Source: CAD feature listing. Evaluate the final solid. Frame: model axes, mm. A direction names the side the tool comes from. Give positions to 0.01 mm unless a question says otherwise; leave off trailing zeros. Write each loop counter-clockwise with the first axis right and the second up, starting at its lowest first coordinate (ties: lowest second). Pieces come first, ordered by that corner, then holes. Notation, with made-up numbers: (42, 51) -> (91, 51) arc R17 cw to (91, 66) -> close; hole circle Ø6 at (1.25, -7.75). An arc over 180 degrees is marked (long way). Use a Markdown table: item, result. Add a question column.
```python
from build123d import *

# Parameters (mm, degrees)
SKETCH_R        = 47.5
SKETCH_R_2      = 1.75
PAD_DEPTH       = 25.65
SKETCH001_R     = 4.5
POCKET_DEPTH    = 7
SKETCH002_R     = 3.1
POCKET001_DEPTH = 25.651
SKETCH003_R     = 6
POCKET002_DEPTH = 7


with BuildPart() as part:
    # Sketch → Pad (new body)
    with BuildSketch(Plane.XY):
        Circle(SKETCH_R)
        with Locations((0, 40.45)):
            Circle(SKETCH_R_2, mode=Mode.SUBTRACT)
        with Locations((-35.05, -20.3)):
            Circle(SKETCH_R_2, mode=Mode.SUBTRACT)
        with Locations((35.05, -20.3)):
            Circle(SKETCH_R_2, mode=Mode.SUBTRACT)
    extrude(amount=PAD_DEPTH)

    # Sketch001 (on Face5 of Pad) → Pocket (cut)
    with BuildSketch(Plane(origin=(0, 0, 0), x_dir=(1, 0, 0), z_dir=(0, 0, -1))):
        with Locations((-35.05, 20.3)):
            Circle(SKETCH001_R)
        with Locations((35.05, 20.3)):
            Circle(SKETCH001_R)
        with Locations((0, -40.45)):
            Circle(SKETCH001_R)
    extrude(amount=-POCKET_DEPTH, mode=Mode.SUBTRACT)

    # Sketch002 (on Face2 of Pocket) → Pocket001 (cut, through all)
    with BuildSketch(Plane(origin=(0, 0, 0), x_dir=(1, 0, 0), z_dir=(0, 0, -1))):
        with Locations((0, 25)):
            Circle(SKETCH002_R)
        with Locations((25, 0)):
            Circle(SKETCH002_R)
        with Locations((-25, 0)):
            Circle(SKETCH002_R)
        with Locations((0, -25)):
            Circle(SKETCH002_R)
    extrude(amount=-POCKET001_DEPTH, mode=Mode.SUBTRACT)

    # Sketch003 (on Face3 of Pocket001) → Pocket002 (cut)
    with BuildSketch(Plane.XY.offset(25.65)):
        with Locations((0, 25)):
            Circle(SKETCH003_R)
        with Locations((0, -25)):
            Circle(SKETCH003_R)
        with Locations((25, 0)):
            Circle(SKETCH003_R)
        with Locations((-25, 0)):
            Circle(SKETCH003_R)
    extrude(amount=-POCKET002_DEPTH, mode=Mode.SUBTRACT)


solid = part.part
```
(1) Cut plane B-B on z = 9.25. Return the cut outline in (x, y), then the cut area to 3 significant figures.
(2) First-contact query: pin 1 Ø3 at (x, z) = (3.5, 19) entering from +Y; pin 2 Ø10 at (y, z) = (36.5, 12) entering from -X; pin 3 Ø5 at (x, z) = (-4, 12) entering from -Y; pin 4 Ø3 at (x, y) = (-35.05, -20.3) entering from -Z. Flat tips, straight axial feed; report the tip coordinate or a pass-through.
(3) Cut plane D-D on y = -23.5. Return the cut outline in (x, z), then the cut area to 3 significant figures.
(4) Access query for faces 1 (the cylindrical face through (-27.46, 1.886, 9.194)), 2 (the cylindrical face through (-29.76, -3.65, 22.2)), 3 (the cylindrical face through (34.46, -24.76, 3.45)). Directions: +Z, -Z, +X, -X, +Y, -Y. A direction counts if a zero-diameter tool reaches every point of the face in a straight line with its end or side. Return the directions, or none.
(5) Cut plane A-A on y = 0. Return the cut outline in (x, z).
(6) Cut plane C-C on x = 25.5. Return the cut outline in (y, z), then the cut area to 3 significant figures.
(7) Material intervals for L1, parallel to Y at x = 0, z = 7.5; L2, parallel to Y at x = 0, z = 19.5; L3, parallel to X at y = 42, z = 19.25, sorted ascending.
(8) Mould query, pull axis X, two halves, no side actions, for faces 4 (the cylindrical face through (-10.3, -46.37, 12.65)), 5 (the cylindrical face through (20.24, -3.65, 22.2)), 6 (the flat face through (-1, 1, 0)). Classes: +X half, -X half, draft (parallel to the pull), parting line (faces both ways), or undercut.
Output:
| question | item | result |
|---|---|---|
| 1 | outline | circle Ø95 at (0, 0); hole circle Ø3.5 at (-35.05, -20.3); hole circle Ø6.2 at (-25, 0); hole circle Ø6.2 at (0, -25); hole circle Ø6.2 at (0, 25); hole circle Ø3.5 at (0, 40.45); hole circle Ø6.2 at (25, 0); hole circle Ø3.5 at (35.05, -20.3) |
| 1 | area | 6,940 mm^2 |
| 2 | pin 1 | y = 47.46 |
| 2 | pin 2 | x = -35.55 |
| 2 | pin 3 | y = -47.48 |
| 2 | pin 4 | through |
| 3 | outline | (-41.28, 0) -> (-38.21, 0) -> (-38.21, 7) -> (-31.89, 7) -> (-31.89, 0) -> (-2.71, 0) -> (-2.71, 18.65) -> (-5.81, 18.65) -> (-5.81, 25.65) -> (-41.28, 25.65) -> close; (2.71, 0) -> (31.89, 0) -> (31.89, 7) -> (38.21, 7) -> (38.21, 0) -> (41.28, 0) -> (41.28, 25.65) -> (5.81, 25.65) -> (5.81, 18.65) -> (2.71, 18.65) -> close |
| 3 | area | 1,850 mm^2 |
| 4 | face 1 | +Z, -Z |
| 4 | face 2 | +Z |
| 4 | face 3 | -Z |
| 5 | outline | (-47.5, 0) -> (-28.1, 0) -> (-28.1, 18.65) -> (-31, 18.65) -> (-31, 25.65) -> (-47.5, 25.65) -> close; (-21.9, 0) -> (21.9, 0) -> (21.9, 18.65) -> (19, 18.65) -> (19, 25.65) -> (-19, 25.65) -> (-19, 18.65) -> (-21.9, 18.65) -> close; (28.1, 0) -> (47.5, 0) -> (47.5, 25.65) -> (31, 25.65) -> (31, 18.65) -> (28.1, 18.65) -> close |
| 6 | outline | (-40.07, 0) -> (-3.06, 0) -> (-3.06, 18.65) -> (-5.98, 18.65) -> (-5.98, 25.65) -> (-40.07, 25.65) -> close; (3.06, 0) -> (40.07, 0) -> (40.07, 25.65) -> (5.98, 25.65) -> (5.98, 18.65) -> (3.06, 18.65) -> close |
| 6 | area | 1,860 mm^2 |
| 7 | L1 | -47.5 to -28.1, -21.9 to 21.9, 28.1 to 38.7, 42.2 to 47.5 |
| 7 | L2 | -47.5 to -31, -19 to 19, 31 to 38.7, 42.2 to 47.5 |
| 7 | L3 | -22.19 to -0.81, 0.81 to 22.19 |
| 8 | face 4 | parting line |
| 8 | face 5 | undercut |
| 8 | face 6 | draft |
